Work out the finished part from the listing and answer in its coordinate system (mm). A direction names the side the tool comes from. Coordinates: 2 decimals unless noted, no trailing zeros. Write each loop counter-clockwise with the first axis right and the second up, starting at its lowest first coordinate (ties: lowest second). Pieces come first, ordered by that corner, then holes. Notation, with made-up numbers: (63, -1) - (78, -1) arc R26 ccw to (78, 38) - close; hole circle Ø2 at (89, 28). An arc over 180 degrees is marked (long way). One line per item, written item: value.
Autodesk Inventor part; units mm, degrees
ref_plane "YZ Plane" through (0, 0, 0) normal (1, 0, 0) x (0, 1, 0)
ref_plane "XZ Plane" through (0, 0, 0) normal (0, 1, 0) x (-1, 0, 0)
ref_plane "XY Plane" through (0, 0, 0) normal (0, 0, 1) x (1, 0, 0)
sketch "Sketch2" plane through (0, 0, 0) normal (0, 0, 1) x (1, 0, 0)
  line L0 (0, -57.05) -> (0, 57.05) construction
  line L1 (-56.66, 0) -> (58.56, 0) construction
  line L2 (-24.5, 0) -> (-24.5, -12.575)
  line L3 (-24.5, -12.575) -> (-40.2, -12.575)
  line L4 (-40.2, -12.575) -> (-40.2, -36.2257)
  line L5 (-40.2, -36.2257) -> (24.5, -40.75)
  line L6 (24.5, -40.75) -> (24.5, -11.75)
  line L7 (24.5, -11.75) -> (42.1, -11.75)
  line L8 (42.1, -11.75) -> (42.1, 0)
  line L9 (-24.5, 0) -> (-24.5, 12.575)
  line L10 (-24.5, 12.575) -> (-40.2, 12.575)
  line L11 (-40.2, 12.575) -> (-40.2, 36.2257)
  line L12 (-40.2, 36.2257) -> (24.5, 40.75)
  line L13 (24.5, 40.75) -> (24.5, 11.75)
  line L14 (24.5, 11.75) -> (42.1, 11.75)
  line L15 (42.1, 11.75) -> (42.1, 0)
  line L16 (-35, 12.575) -> (-35, -12.575) construction
  line L17 (35, 11.75) -> (35, -11.75) construction
  point P0 (0, 0)
  dimension "d0" = 25.15
  dimension "d1" = 70
  dimension "d2" = 10.5
  dimension "d3" = 10.5
  dimension "d4" = 5.2
  dimension "d5" = 7.1
  dimension "d6" = 23.5
  dimension "d7" = 81.5
  dimension "d8" = 8
extrude "Extrusion1" add sketch "Sketch2" along normal blind 3
fillet "Fillet1" [suppressed]
sketch "Sketch3" plane through (0, 0, 3) normal (0, 0, 1) x (1, 0, 0)
  line L0 (-30.15, -25.625) -> (24.5, -25.625) construction
  line L1 (24.5, -40.75) -> (24.5, -11.75) construction
  line L2 (-40.2, -36.2257) -> (24.5, -40.75) construction
  line L3 (-40.2, -12.575) -> (-40.2, -36.2257) construction
  line L4 (-24.5, -12.575) -> (-40.2, -12.575) construction
  line L5 (24.5, -12.75) -> (-30.15, -12.75)
  line L6 (-30.15, -12.75) -> (-30.15, -36.9285)
  line L7 (-30.15, -36.9285) -> (24.5, -40.75)
  line L8 (24.5, -12.75) -> (24.5, -40.75)
  point P0 (0, 0)
  dimension "d12" = 25.625
  dimension "d13" = 28
  dimension "d14" = 54.65
extrude "Extrusion2" add sketch "Sketch3" along normal blind 19
sketch "Sketch4" plane through (0, 0, 22) normal (0, 0, 1) x (1, 0, 0)
  line L0 (-30.15, -25.625) -> (24.5, -25.625) construction
  line L1 (-30.15, -36.9285) -> (24.5, -40.75) construction
  line L2 (-30.15, -12.75) -> (-30.15, -36.9285)
  line L3 (24.5, -40.75) -> (24.5, -12.75)
  line L4 (-30.15, -25.625) -> (24.5, -25.625)
  line L5 (-30.15, -36.9285) -> (-30.15, -37.2292)
  line L6 (-30.15, -37.2292) -> (24.5, -41.0507)
  line L7 (24.5, -41.0507) -> (24.5, -40.75)
  point P0 (0, 0)
  dimension "d18" = 0.3
revolve "Revolution1" cut sketch "Sketch4" angle 360 about axis through (-30.15, -25.625, 22) along (1, 0, 0)
mirror "Mirror1" about plane through (0, 0, 0) normal (0, 1, 0) of "Extrusion2", "Revolution1"
equation "\"d0\" = finger_width + 2 * finger_link_clearence"
equation "\"finger_width\" = 25"
equation "\"finger_thickness\" = 8"
equation "\"finger_part_A_length\" = 42.8625"
equation "\"finger_part_B_length\" = 28.575"
equation "\"finger_link_width\" = 3.5"
equation "\"finger_link_clearence\" = 0.075"
equation "\"tol\" = 0.5 * finger_link_clearence"
equation "\"link_tol\" = 0.254"
equation "\"bore_press\" = 2.925"
equation "\"bore_clearance\" = 3.025"
equation "\"bar_diameter\" = 6.5"
equation "\"bar_thickness\" = 4"
equation "\"bar_width\" = 7"
equation "\"hinge_dist_sym_plane\" = 4"
equation "\"hinge_thickness\" = 3"
equation "\"hinge_act_length_c\" = 7.62"
equation "\"hinge_act_length_bc\" = 16.66875"
equation "\"hinge_act_length_ab\" = 11.049"
equation "\"hinge_act_length_a\" = 21.43125"
equation "\"hinge_guid_length_c\" = 9.525"
equation "\"hinge_guid_length_bc\" = 9.525"
equation "\"hinge_guid_length_ab\" = 17.145"
equation "\"hinge_guid_length_a\" = 17.145"
equation "\"bar_length_bc\" = finger_part_B_length"
equation "\"bar_act_length_ab\" = 40.48125"
equation "\"bar_guid_length_ab\" = 43.275"
equation "\"champfer\" = 0.3"
equation "\"fillet\" = 0.4"
equation "\"gear_diameter\" = 14"
equation "\"dist_finger_BC\" = 56.5"
equation "\"hinge_point\" = 15"
properties part number "hand-palm"
Item 1: Given pin 1 (4 mm diameter, centred on y = -21, z = 6.5, fed in from -X); pin 2 (1.1 mm diameter, centred on x = 6.5, y = 38.5, fed in from -Z); pin 3 (1.5 mm diameter, centred on x = 7.5, z = 7.5, fed in from +Y); pin 4 (1 mm diameter, centred on x = -11.5, z = 8.5, fed in from -Y), each flat-ended and moving along its own axis, determine where each tip first touches the part or whether it passes through.
Evaluation:
pin 1: stops at x = -30.15
pin 2: stops at z = 0
pin 3: stops at y = 39.61
pin 4: stops at y = -38.27
Item 2: Determine the mould class of faces 1 (the face through (-2.442, 38.866, 11.073)), 2 (the face through (-24.5, 0, 1)), 3 (the face through (33, -11.75, 1)) for opening direction Y: +Y half, -Y half, draft (parallel to the pull), parting line (faces both ways), or undercut.
Evaluation:
face 1: +Y half
face 2: undercut
face 3: -Y half
Item 3: Consider probe 1 along X at (y, z) = (-32.5, 4.75); probe 2 along Y at (x, z) = (-32, 2.5) (3 decimals); probe 3 along Y at (x, z) = (-30, 1.25) (3 decimals). Determine where each line is inside the solid, lowest interval first.
Evaluation:
probe 1: x = -30.15 to 24.5
probe 2: y = -36.799 to -12.575, 12.575 to 36.799
probe 3: y = -36.939 to -12.575, 12.575 to 36.939
Item 4: Which of the six approach directions +Z, -Z, +X, -X, +Y, -Y give full straight-line access (tool end or side, diameter ignored) to faces 4 (the face through (24.5, -26, 5)), 5 (the face through (33, 11.75, 1)), 6 (the face through (-3, 12.75, 10)), 7 (the face through (-32, 12.575, 1)), 8 (the face through (-2, 0, 3))?
Evaluation:
face 4: +Z, -Z, +X, -Y
face 5: +Z, -Z, +X, +Y
face 6: +Z, +X, -X
face 7: +Z, -Z, -X
face 8: +Z, -X
Item 5: Section A-A, the plane z = 4.5 is taken. Determine the outline of the cut face in (x, y).
Evaluation:
outline: (-30.15, -36.93) - (24.5, -40.75) - (24.5, -12.75) - (-30.15, -12.75) - close; (-30.15, 12.75) - (24.5, 12.75) - (24.5, 40.75) - (-30.15, 36.93) - close
Item 6: Section C-C, the plane y = -2.5 is taken. Determine the outline of the cut face in (x, z).
Evaluation:
outline: (-24.5, 0) - (42.1, 0) - (42.1, 3) - (-24.5, 3) - close
Item 7: Section D-D, the plane z = 11.75 is taken. Give the number of separate pieces and of enclosed holes in the cut face, then the cut area to 3 significant figures.
Evaluation:
separate pieces: 4
enclosed holes: 0
area: 948 mm2
